Geometry: see drawing. Coordinates: mm, zero at the bounding-box minimum. A direction names the side the tool comes from. Coordinates: 2 decimals unless noted, no trailing zeros. Order: outer loops, then holes, each group sorted by start corner. A loop starts at its lowest first (then second) coordinate and runs counter-clockwise, first axis right, second up. Notation, with made-up numbers: (45, 75.25) -> (60, 75.25) arc R26 ccw to (60, 100.25) -> close; hole circle Ø4 at (15.25, 2.25). An arc over 180 degrees is marked (long way). Write each question's results on one line, items separated by ' | '.
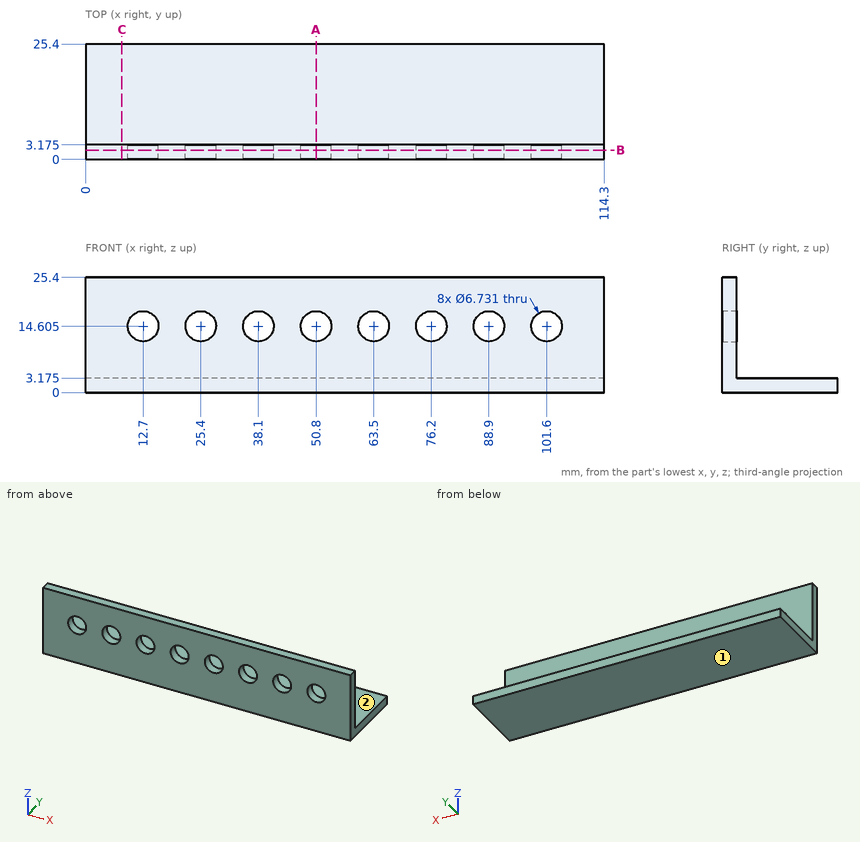
(1) Line query: line 1 along Z through (x, y) = (76.2, 1.4); line 2 along Y through (x, z) = (61, 5.5) (3 decimals). Output: solid intervals per line, ascending. Write a range as from..to.
Return value:
line 1: 0..11.24, 17.97..25.4 | line 2: 0..3.175
(2) Cut plane B-B, the plane y = 2. Count the separate pieces of the cut face and the enclosed holes in it, plus the area to 3 significant figures.
Return value:
separate pieces: 1 | enclosed holes: 8 | area: 2,620 mm2
(3) Cut plane A-A, the plane x = 50.8. Return loops of the section in (y, z) (1 decimal).
Return value:
outline: (0, 0) -> (25.4, 0) -> (25.4, 3.2) -> (3.2, 3.2) -> (3.2, 11.2) -> (0, 11.2) -> close; (0, 18) -> (3.2, 18) -> (3.2, 25.4) -> (0, 25.4) -> close
(4) Reachability of the marked faces 1 and 2 from +Z, -Z, +X, -X, +Y, -Y: full face, straight path, thin tool, end or side. Return the list, or none.
Return value:
face 1: -Z, +X, -X, +Y, -Y | face 2: +Z, +X, -X, +Y
(5) Cut plane C-C, the plane x = 8. Return loops of the section in (y, z) (3 decimals).
Return value:
outline: (0, 0) -> (25.4, 0) -> (25.4, 3.175) -> (3.175, 3.175) -> (3.175, 25.4) -> (0, 25.4) -> close
(6) Pin query (flat end, axial travel): P1, Ø4, axis at x = 38.1, z = 14.605, coming from the +Y side; P2, Ø3, axis at x = 87, y = 20.5, coming from the -Z side; P3, Ø6, axis at x = 73.5, y = 14.5, coming from the +Z side (3 decimals); P4, Ø9, axis at x = 63.5, z = 14.605, coming from the +Y side (3 decimals). Return the tip coordinate at first contact, or that it passes through.
Return value:
P1: through | P2: z = 0 | P3: z = 3.175 | P4: y = 3.175
